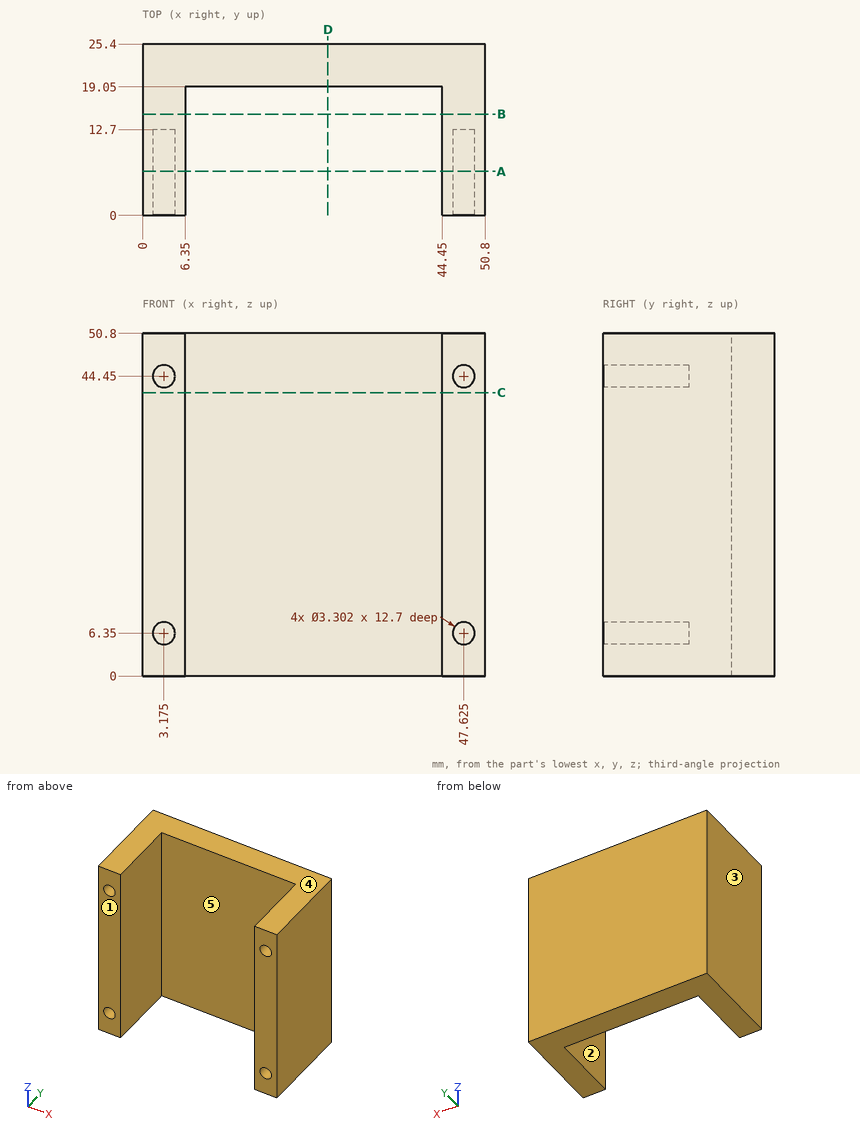
Check sheet for the drawn part. Datum: minimum x, y, z corner. Units: mm. A direction names the side the tool comes from. Round coordinates to 2 decimals unless told otherwise and drop trailing zeros. Loops run counter-clockwise (first coordinate to the right, second up) from the corner with the lowest first, then second, coordinate; pieces in that order, holes last.
Item 1: Gauge pin test, flat ends, axial feed: pin 1 (1 mm diameter, centred on x = 3.5, z = 6.5, fed in from -Y); pin 2 (5 mm diameter, centred on x = 12.5, z = 23.5, fed in from -Y). Record the tip position at first contact, or that the pin passes through.
Item 2: Cross-section at C-C on z = 42. Record the boundary of the cut face in (x, y), then the cut area to 3 significant figures.
Item 3: Cross-section at A-A on y = 6.5. Record the boundary of the cut face in (x, z) (3 decimals), then the cut area to 3 significant figures.
Item 4: Access from +Z, -Z, +X, -X, +Y, -Y to the whole of each face (thin tool, end or side, straight path). Record for the marked faces 4 and 5.
Item 5: Thickness scan on line 1 (Z direction, x = 3, y = 5); line 2 (X direction, y = 15.5, z = 44); line 3 (X direction, y = 4.75, z = 43). Record the ranges inside material, lowest first.
Item 6: Mould release check, pull along X, two halves, no side actions. Record for the marked faces 1, 2 and 3: pulls with the +X half, pulls with the -X half, needs draft (parallel to the pull), parting line crosses it, or undercut.
Item 7: Cross-section at D-D on x = 27.5. Record the boundary of the cut face in (y, z).
Item 8: Cross-section at B-B on y = 15. Record the boundary of the cut face in (x, z), then the cut area to 3 significant figures.
Answer sheet:
1. pin 1: stops at y = 12.7
1. pin 2: stops at y = 19.05
2. outline: (0, 0) - (6.35, 0) - (6.35, 19.05) - (44.45, 19.05) - (44.45, 0) - (50.8, 0) - (50.8, 25.4) - (0, 25.4) - close
2. area: 565 mm2
3. outline: (0, 0) - (6.35, 0) - (6.35, 50.8) - (0, 50.8) - close; (44.45, 0) - (50.8, 0) - (50.8, 50.8) - (44.45, 50.8) - close; hole circle Ø3.302 at (3.175, 6.35); hole circle Ø3.302 at (3.175, 44.45); hole circle Ø3.302 at (47.625, 6.35); hole circle Ø3.302 at (47.625, 44.45)
3. area: 611 mm2
4. face 4: +Z, +X, -X, +Y, -Y
4. face 5: +Z, -Z, -Y
5. line 1: z = 0 to 4.71, 7.99 to 42.81, 46.09 to 50.8
5. line 2: x = 0 to 6.35, 44.45 to 50.8
5. line 3: x = 0 to 2.39, 3.96 to 6.35, 44.45 to 46.84, 48.41 to 50.8
6. face 1: needs draft
6. face 2: undercut
6. face 3: pulls with the -X half
7. outline: (19.05, 0) - (25.4, 0) - (25.4, 50.8) - (19.05, 50.8) - close
8. outline: (0, 0) - (6.35, 0) - (6.35, 50.8) - (0, 50.8) - close; (44.45, 0) - (50.8, 0) - (50.8, 50.8) - (44.45, 50.8) - close
8. area: 645 mm2
